Source: three-view drawing plus pictorial views. Frame: mm from the lowest corner of the part. Give positions to 0.01 mm unless a question says otherwise; leave off trailing zeros. Loops run counter-clockwise (first coordinate to the right, second up) from the corner with the lowest first, then second, coordinate; pieces in that order, holes last.
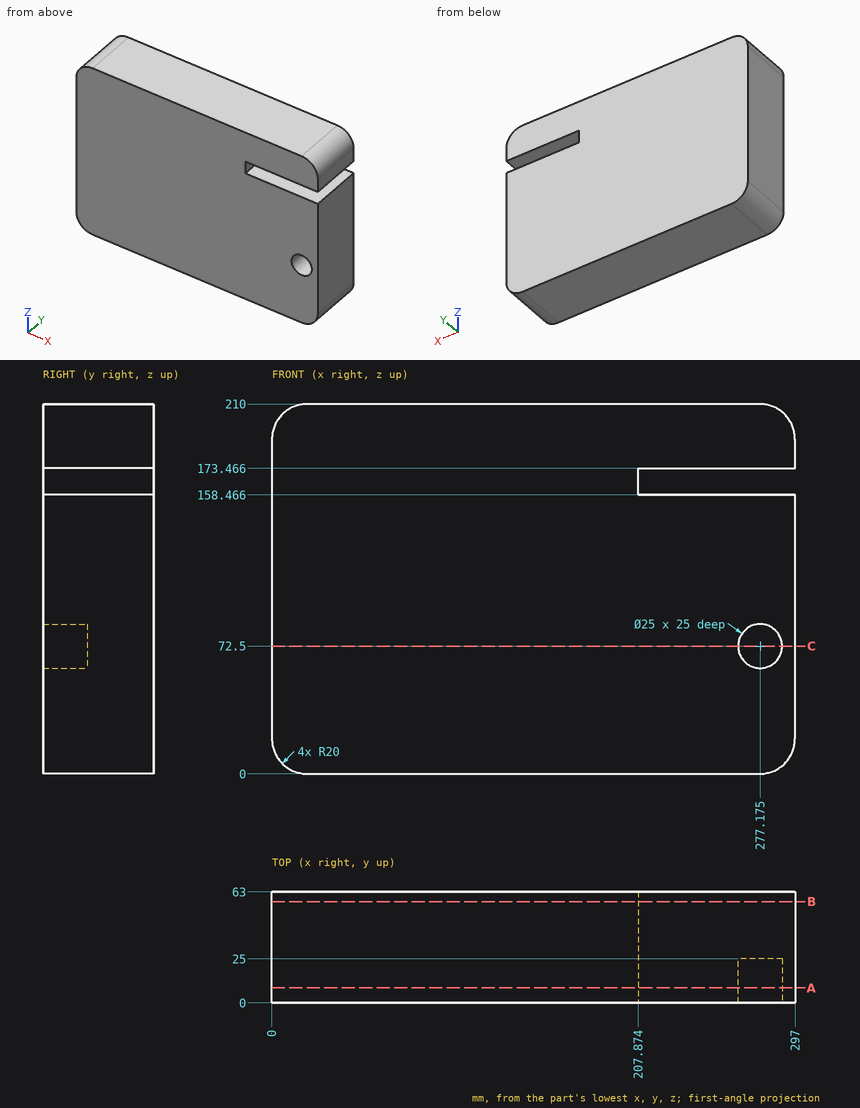
(1) Cut plane C-C (z = 72.5). Return the cut outline in (x, y) (1 decimal).
Values follow:
outline: (0, 0) - (264.7, 0) - (264.7, 25) - (289.7, 25) - (289.7, 0) - (297, 0) - (297, 63) - (0, 63) - close
(2) Ray query, probe 1 along Z at (x, y) = (222, 23); probe 2 along X at (y, z) = (8, 72) (1 decimal); probe 3 along X at (y, z) = (29, 168) (1 decimal). Return the intervals inside material, ascending.
Values follow:
probe 1: z = 0 to 158.47, 173.47 to 210
probe 2: x = 0 to 264.7, 289.7 to 297
probe 3: x = 0 to 207.9
(3) Cut plane B-B (y = 57.5). Return the cut outline in (x, z) (1 decimal).
Values follow:
outline: (0, 20) arc R20 ccw to (20, 0) - (277, 0) arc R20 ccw to (297, 20) - (297, 158.5) - (207.9, 158.5) - (207.9, 173.5) - (297, 173.5) - (297, 190) arc R20 ccw to (277, 210) - (20, 210) arc R20 ccw to (0, 190) - close
(4) Cut plane A-A (y = 8.5). Return the cut outline in (x, z) (1 decimal), and give its area (3 significant figures).
Values follow:
outline: (0, 20) arc R20 ccw to (20, 0) - (277, 0) arc R20 ccw to (297, 20) - (297, 158.5) - (207.9, 158.5) - (207.9, 173.5) - (297, 173.5) - (297, 190) arc R20 ccw to (277, 210) - (20, 210) arc R20 ccw to (0, 190) - close; hole circle Ø25 at (277.2, 72.5)
area: 60,200 mm2
(5) Pin query (flat end, axial travel): pin 1 Ø12.5 at (x, z) = (278.5, 66.5) entering from -Y. Return the tip coordinate at first contact, or that it passes through.
Values follow:
pin 1: stops at y = 25
